from build123d import *

# Parameters (mm, degrees)
F1_DEPTH = 15
F3_D     = 6.6
F4_SIZE2 = 2
F4_SIZE  = 2


with BuildPart() as f1:
    # F0 (on Top) → F1 (new body)
    with BuildSketch(Plane.XY):
        with BuildLine():
            ThreePointArc((7.483315, -0.5), (0, -7.5), (-7.483315, -0.5))
            Line((-7.483315, -0.5), (-27.5, -0.5))
            Line((-27.5, -0.5), (-27.5, -15.5))
            Line((-27.5, -15.5), (27.5, -15.5))
            Line((27.5, -15.5), (27.5, -0.5))
            Line((27.5, -0.5), (7.483315, -0.5))
        make_face()
    extrude(amount=F1_DEPTH)

    # F3 (through all)
    with Locations(Plane(origin=(0, -0.5, 0), x_dir=(-1, 0, 0), z_dir=(0, 1, 0))):
        with Locations((17.491657, 7.5), (-17.491657, 7.5)):
            Hole(F3_D / 2)

    # F4
    f4_edges = [f1.edges().sort_by_distance(p)[0] for p in [
        (-27.5, -15.5, 7.5),
        (27.5, -15.5, 7.5),
    ]]
    chamfer(f4_edges, length=F4_SIZE, length2=F4_SIZE2)


solid = f1.part
Model file for the job. Use its own axes, mm. Coordinates: 2 decimals unless noted, no trailing zeros. Write each loop counter-clockwise with the first axis right and the second up, starting at its lowest first coordinate (ties: lowest second). Pieces come first, ordered by that corner, then holes. Notation, with made-up numbers: (25.25, 39.5) -> (55.25, 39.5) arc R24 cw to (55.25, 55.5) -> close; hole circle Ø4 at (-5, 40). An arc over 180 degrees is marked (long way). One line per item, written item: value. Start each with the question number.
1) Slice it at C-C on y = -14.5. Write the cut outline in (x, z), then the cut area to 3 significant figures.
2) Slice it at B-B on y = -4.25. Write the cut outline in (x, z), then the cut area to 3 significant figures.
3) Probe probe 1 along X at (y, z) = (-14.25, 10); probe 2 along Y at (x, z) = (0, 10.75); probe 3 along X at (y, z) = (-7.75, 9). List the from-to ranges inside material, lowest first.
4) Pull direction X, two halves, no side cores. Call faces 1 (the face through (0, -8, 15)), 2 (the face through (26, -15, 7)), 3 (the face through (-20.79, -8.11, 7.65)), 4 (the face through (20.54, -8.11, 6.24)): +X half, -X half, draft (parallel to the pull), parting line (faces both ways), or undercut.
5) Slice it at D-D on z = 2.5. Write the cut outline in (x, y).
6) Slice it at A-A on z = 7.5. Write the cut outline in (x, y).
Answers follow:
1. outline: (-26.5, 0) -> (26.5, 0) -> (26.5, 15) -> (-26.5, 15) -> close; hole circle Ø6.6 at (-17.49, 7.5); hole circle Ø6.6 at (17.49, 7.5)
1. area: 727 mm2
2. outline: (-27.5, 0) -> (-6.18, 0) -> (-6.18, 15) -> (-27.5, 15) -> close; (6.18, 0) -> (27.5, 0) -> (27.5, 15) -> (6.18, 15) -> close; hole circle Ø6.6 at (-17.49, 7.5); hole circle Ø6.6 at (17.49, 7.5)
2. area: 571 mm2
3. probe 1: -26.75 to -19.65, -15.34 to 15.34, 19.65 to 26.75
3. probe 2: -15.5 to -7.5
3. probe 3: -27.5 to -20.43, -14.55 to 14.55, 20.43 to 27.5
4. face 1: draft
4. face 2: +X half
4. face 3: undercut
4. face 4: undercut
5. outline: (-27.5, -13.5) -> (-25.5, -15.5) -> (25.5, -15.5) -> (27.5, -13.5) -> (27.5, -0.5) -> (7.48, -0.5) arc R7.5 cw to (-7.48, -0.5) -> (-27.5, -0.5) -> close
6. outline: (-27.5, -13.5) -> (-25.5, -15.5) -> (-20.79, -15.5) -> (-20.79, -0.5) -> (-27.5, -0.5) -> close; (-14.19, -15.5) -> (14.19, -15.5) -> (14.19, -0.5) -> (7.48, -0.5) arc R7.5 cw to (-7.48, -0.5) -> (-14.19, -0.5) -> close; (20.79, -15.5) -> (25.5, -15.5) -> (27.5, -13.5) -> (27.5, -0.5) -> (20.79, -0.5) -> close
